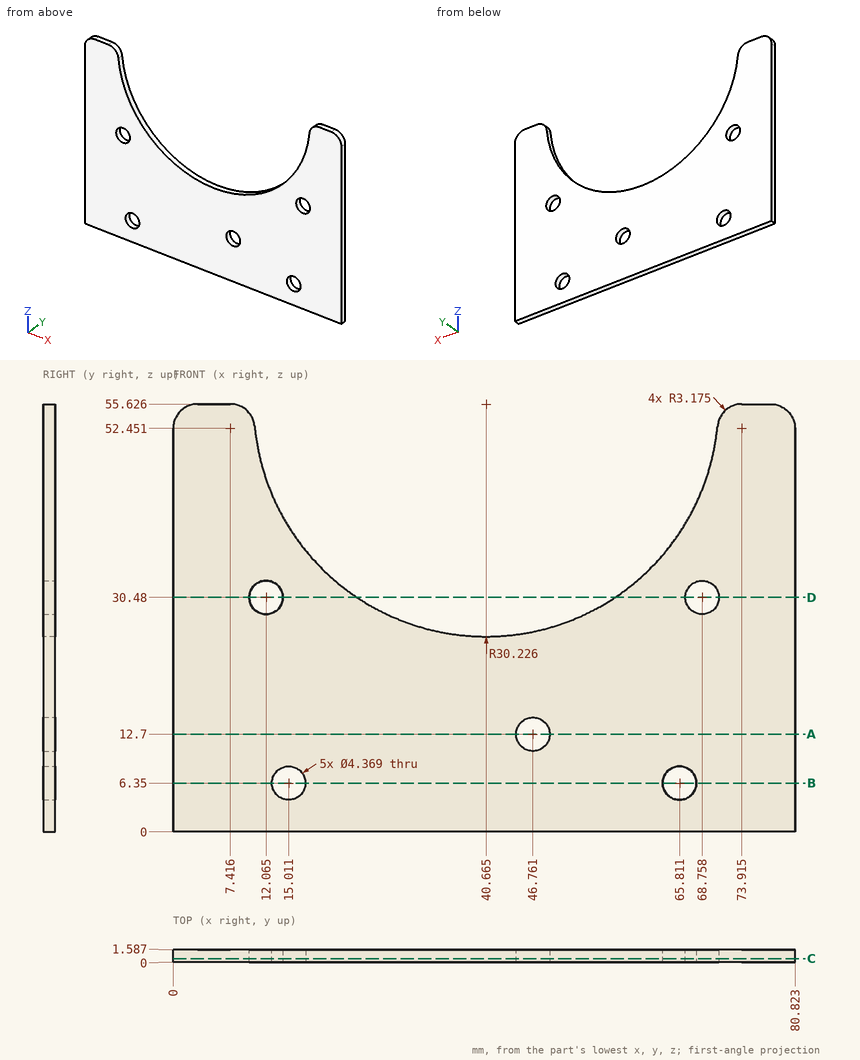
Check sheet for the drawn part. Datum: minimum x, y, z corner. Units: mm. Give positions to 0.01 mm unless a question says otherwise; leave off trailing zeros. Write each loop counter-clockwise with the first axis right and the second up, starting at its lowest first coordinate (ties: lowest second). Pieces come first, ordered by that corner, then holes. Notation, with made-up numbers: (14.5, -26) -> (31.5, -26) arc R13 ccw to (31.5, -2) -> close; hole circle Ø6 at (24.5, 30.25). An arc over 180 degrees is marked (long way). Use one line per item in the form item = value. Start each with the question number.
1. Section check D-D (z = 30.48). Record the cut outline in (x, y).
2. Section check C-C (y = 0.45). Count the separate pieces of the cut face and the enclosed holes in it, and give its area (3 significant figures).
3. Section check A-A (z = 12.7). Record the cut outline in (x, y) (1 decimal).
4. Section check B-B (z = 6.35). Record the cut outline in (x, y) (1 decimal).
5. Thickness scan on line 1 along X through (y, z) = (0.45, 12.5) (1 decimal); line 2 along X through (y, z) = (0.9, 8) (1 decimal); line 3 along X through (y, z) = (1.25, 41.5) (1 decimal). Record the ranges inside material, lowest first. Write a range as from..to.
Conclusion:
q1.outline = (0, 0) -> (9.88, 0) -> (9.88, 1.59) -> (0, 1.59) -> close; (14.25, 0) -> (23.89, 0) -> (23.89, 1.59) -> (14.25, 1.59) -> close; (57.44, 0) -> (66.57, 0) -> (66.57, 1.59) -> (57.44, 1.59) -> close; (70.94, 0) -> (80.82, 0) -> (80.82, 1.59) -> (70.94, 1.59) -> close
q2.separate_pieces = 1
q2.enclosed_holes = 5
q2.area = 2,980 mm²
q3.outline = (0, 0) -> (44.6, 0) -> (44.6, 1.6) -> (0, 1.6) -> close; (48.9, 0) -> (80.8, 0) -> (80.8, 1.6) -> (48.9, 1.6) -> close
q4.outline = (0, 0) -> (12.8, 0) -> (12.8, 1.6) -> (0, 1.6) -> close; (17.2, 0) -> (63.6, 0) -> (63.6, 1.6) -> (17.2, 1.6) -> close; (68, 0) -> (80.8, 0) -> (80.8, 1.6) -> (68, 1.6) -> close
q5.line_1 = 0..44.6, 48.9..80.8
q5.line_2 = 0..13.6, 16.4..64.4, 67.2..80.8
q5.line_3 = 0..13.9, 67.4..80.8
